```python
from build123d import *

# Parameters (mm, degrees)
SKETCH_1_R               = 8.5
SKETCH_1_R_2             = 4.5
SKETCH_1_R_3             = 3
SKETCH_1_R_4             = 1.4
EXTRUDE_1_DEPTH          = 3
FILLET_1_R               = 2
SKETCH_2_R               = 3
EXTRUDE_2_DEPTH          = 7
EXTRUDE_2_DEPTH_BACK     = 3
SKETCH_3_R               = 1.4
CUT_EXTRUDE_1_DEPTH      = 1
CUT_EXTRUDE_1_DEPTH_BACK = 11


with BuildPart() as part:
    # Эскиз1 → Бобышка-Вытянуть1 (new body)
    with BuildSketch(Plane(origin=(0, 0, 0), x_dir=(1, 0, 0), z_dir=(0, 1, 0))):
        Polygon((8.15, -20), (8.15, -12.25), (23.75, -3.757292419), (23.75, 24.742707581), (4.725, 35.1), (-4.725, 35.1), (-23.75, 24.742707581), (-23.75, -3.757292419), (-8.15, -12.25), (-8.15, -20), align=None)
        Circle(SKETCH_1_R, mode=Mode.SUBTRACT)
        with Locations((-9.5, 14.5)):
            Circle(SKETCH_1_R_2, mode=Mode.SUBTRACT)
        with Locations((3.53, 20.8)):
            Circle(SKETCH_1_R_3, mode=Mode.SUBTRACT)
        with Locations((12.43, 20.8)):
            Circle(SKETCH_1_R_3, mode=Mode.SUBTRACT)
        with Locations((19.54, 19.1)):
            Circle(SKETCH_1_R_4, mode=Mode.SUBTRACT)
        with Locations((19.54, 9.5)):
            Circle(SKETCH_1_R_4, mode=Mode.SUBTRACT)
        with Locations((-19.54, 19.1)):
            Circle(SKETCH_1_R_4, mode=Mode.SUBTRACT)
        with Locations((-19.54, 9.5)):
            Circle(SKETCH_1_R_4, mode=Mode.SUBTRACT)
        with Locations((0, 29.1)):
            Circle(SKETCH_1_R_4, mode=Mode.SUBTRACT)
    extrude(amount=EXTRUDE_1_DEPTH)

    # Скругление1
    fillet_1_edges = [part.edges().sort_by_distance(p)[0] for p in [
        (-8.15, 1.5, 20),
        (-8.15, 1.5, 12.25),
        (-23.75, 1.5, 3.757292419),
        (-23.75, 1.5, -24.742707581),
        (-4.725, 1.5, -35.1),
        (4.725, 1.5, -35.1),
        (23.75, 1.5, -24.742707581),
        (23.75, 1.5, 3.757292419),
        (8.15, 1.5, 12.25),
        (8.15, 1.5, 20),
    ]]
    fillet(fillet_1_edges, radius=FILLET_1_R)

    # Эскиз2 → Бобышка-Вытянуть2 (add, two sides)
    with BuildSketch(Plane(origin=(0, 3, 0), x_dir=(1, 0, 0), z_dir=(0, 1, 0))) as extrude_2_sk:
        with Locations((0, -18.5)):
            Circle(SKETCH_2_R)
        with BuildLine():
            Line((-1.949769217, 7.22), (1.949769217, 7.22))
            ThreePointArc((1.949769217, 7.22), (0, 12.5), (-1.949769217, 7.22))
        make_face()
    extrude(amount=EXTRUDE_2_DEPTH)
    extrude(extrude_2_sk.sketch, amount=-EXTRUDE_2_DEPTH_BACK)

    # Эскиз3 → Вырез-Вытянуть1 (cut, two sides)
    with BuildSketch(Plane(origin=(0, 10, 0), x_dir=(1, 0, 0), z_dir=(0, 1, 0))) as cut_extrude_1_sk:
        with Locations((0, 9.5)):
            Circle(SKETCH_3_R)
        with Locations((0, -18.5)):
            Circle(SKETCH_3_R)
    extrude(amount=CUT_EXTRUDE_1_DEPTH, mode=Mode.SUBTRACT)
    extrude(cut_extrude_1_sk.sketch, amount=-CUT_EXTRUDE_1_DEPTH_BACK, mode=Mode.SUBTRACT)


solid = part.part
```
Check sheet for the modelled part. Datum: model origin and axes. Units: mm. A direction names the side the tool comes from. Coordinates: 2 decimals unless noted, no trailing zeros. Order: outer loops, then holes, each group sorted by start corner. A loop starts at its lowest first (then second) coordinate and runs counter-clockwise, first axis right, second up. Notation, with made-up numbers: M 24.25,3 L 36.25,3 A20 cw 36.25,29 Z; hole C 79,-6 d4. An arc over 180 degrees is marked long. Write each question's results on one line, items separated by ' | '. Start each with the question number.
1. Cross-section at C-C on x = -10.5. Record the cut outline in (y, z).
2. Cross-section at D-D on x = 19.54. Record the cut outline in (y, z).
3. Cross-section at A-A on z = -14.5. Record the cut outline in (x, y), and give its area (4 significant figures).
4. Access from +Z, -Z, +X, -X, +Y, -Y to the whole of each face (thin tool, end or side, straight path). Record for faces 1 (the face through (8.15, 1, 16)), 2 (the face through (-4, 1, 20)), 3 (the face through (14.04, 1.48, -23.33)).
5. Material ranges on probe 1 along Z at (x, y) = (0, 7.5); probe 2 along X at (y, z) = (1.65, -9.5); probe 3 along Z at (x, y) = (19.54, 1.5), recorded low to high.
6. Go/stop test with flat-tipped pins: P1, Ø1.5, axis at y = 2, z = 16, coming from the +X side; P2, Ø6, axis at x = 5.5, y = 3.5, coming from the +Z side; P3, Ø3.5, axis at x = -3.5, y = 1.5, coming from the +Z side; P4, Ø24, axis at x = 6.5, z = 3.5, coming from the +Y side. Record where each tip stops, or that it passes through.
7. Cross-section at B-B on y = 5.5. Record the cut outline in (x, z).
8. Mould release check, pull along Z, two halves, no side actions. Record for faces 4 (the face through (-0.303, 5.07, 19.867)), 5 (the face through (23.462, 1.521, 3.603)), 6 (the face through (23.48, 1.52, -24.56)), 7 (the face through (-23.75, 1, -11)): +Z half, -Z half, draft (parallel to the pull), parting line (faces both ways), or undercut.
Checks:
1) outline: M 0,-31.96 L 3,-31.96 L 3,-18.89 L 0,-18.89 Z; M 0,-10.11 L 3,-10.11 L 3,10.97 L 0,10.97 Z
2) outline: M 0,-27.03 L 3,-27.03 L 3,-20.5 L 0,-20.5 Z; M 0,-17.7 L 3,-17.7 L 3,-10.9 L 0,-10.9 Z; M 0,-8.1 L 3,-8.1 L 3,6.05 L 0,6.05 Z
3) outline: M -23.75,0 L -14,0 L -14,3 L -23.75,3 Z; M -5,0 L 23.75,0 L 23.75,3 L -5,3 Z | area: 115.5 mm²
4) face 1: +Z, +X, +Y, -Y | face 2: +Z, -X, +Y, -Y | face 3: +Y, -Y
5) probe 1: z = -12.5 to -10.9, -8.1 to -7.22, 15.5 to 17.1, 19.9 to 21.5 | probe 2: x = -23.75 to -20.94, -18.14 to -1.4, 1.4 to 18.14, 20.94 to 23.75 | probe 3: z = -27.03 to -20.5, -17.7 to -10.9, -8.1 to 6.05
6) P1: stops at x = 8.15 | P2: stops at z = 20.16 | P3: stops at z = 20.94 | P4: stops at y = 10
7) outline: C 0,18.5 d6; M -1.95,-7.22 A3 ccw long 1.95,-7.22 Z; hole C 0,-9.5 d2.8; hole C 0,18.5 d2.8
8) face 4: undercut | face 5: +Z half | face 6: -Z half | face 7: draft
